Autodesk Inventor part; units mm, degrees
ref_plane "YZ Plane" through (0, 0, 0) normal (1, 0, 0) x (0, 1, 0)
ref_plane "XZ Plane" through (0, 0, 0) normal (0, 1, 0) x (-1, 0, 0)
ref_plane "XY Plane" through (0, 0, 0) normal (0, 0, 1) x (1, 0, 0)
sketch "Sketch1" plane through (0, 0, 0) normal (1, 0, 0) x (0, 1, 0)
  line L0 (-8.7654, 33.1522) -> (-8.7039, 33.1268)
  line L1 (8.7039, 33.1268) -> (8.7654, 33.1522)
  line L2 (-5, 27.5835) -> (-5, 0)
  line L3 (5, 27.5835) -> (5, 0)
  arc A0 (-5, 27.5835) -> (-8.7039, 33.1268) centre (-11, 27.5835) ccw
  arc A1 (8.7039, 33.1268) -> (5, 27.5835) centre (11, 27.5835) ccw
  line L4 (-7, 36) -> (7, 36)
  line L5 (-10, 36) -> (-10, 35)
  line L6 (10, 36) -> (10, 35)
  circle A2 centre (0, 0) radius 46 construction
  arc A3 (-10, 35) -> (-8.7654, 33.1522) centre (-8, 35) ccw
  arc A4 (8.7654, 33.1522) -> (10, 35) centre (8, 35) ccw
  circle A5 centre (0, 0) radius 1.5
  arc A6 (-5, 0) -> (5, 0) centre (0, 0) ccw
  line L7 (0, 0) -> (0, 36) construction
  line L8 (-10, 36) -> (-9.7321, 36)
  line L9 (10, 42) -> (-10, 42)
  line L10 (-10, 42) -> (-10, 36)
  line L11 (10, 36) -> (9.7321, 36)
  line L12 (10, 42) -> (10, 36)
  line L13 (-7, 36) -> (-7, 39)
  line L14 (-7, 39) -> (7, 39)
  line L15 (7, 39) -> (7, 36)
  point P0 (-5, 31.5926)
  point P1 (5, 31.5926)
  dimension "d25" = 10
  dimension "d32" = 6
  dimension "d33" = 6
  dimension "d82" = 46
  dimension "d90" = 2
  dimension "d93" = 1
  dimension "d95" = 22.5
  dimension "d109" = 3
  dimension "d112" = 36
  dimension "d113" = 5
  dimension "d115" = 20
  dimension "d118" = 6
  dimension "d120" = 6
extrude "Extrusion10" add sketch "Sketch1" along normal blind 3
fillet "Fillet1" radius 2 2 edges at (1.5, -10, 42) (1.5, 10, 42)
properties part number "27030914CameraMountA-2"
Input: part model. Units: mm. Frame: model coordinates. A direction names the side the tool comes from. Give positions to 0.01 mm unless a question says otherwise; leave off trailing zeros. Order: outer loops, then holes, each group sorted by start corner. A loop starts at its lowest first (then second) coordinate and runs counter-clockwise, first axis right, second up.
1. Section C-C on z = 7. Return the cut outline in (x, y).
Derived:
outline: (0, -5) - (3, -5) - (3, 5) - (0, 5) - close
2. Reachability of faces 1 (the flat face through (1, 0, 36)), 2 (the flat face through (1, 10, 38)), 3 (the flat face through (1, 5, 14)), 4 (the flat face through (1, -5, 14)) from +Z, -Z, +X, -X, +Y, -Y: full face, straight path, thin tool, end or side. Return the list, or none.
Derived:
face 1: +X, -X
face 2: +Z, -Z, +X, -X, +Y
face 3: -Z, +X, -X, +Y
face 4: -Z, +X, -X, -Y
3. Material intervals for L1, parallel to Z at x = 2.15, y = 0; L2, parallel to Y at x = 1.75, z = 27; L3, parallel to Y at x = 2, z = 34, sorted ascending.
Derived:
L1: z = -5 to -1.5, 1.5 to 36, 39 to 42
L2: y = -5 to 5
L3: y = -9.73 to 9.73
4. Section D-D on y = 7.5. Return the cut outline in (x, z).
Derived:
outline: (0, 32.46) - (3, 32.46) - (3, 42) - (0, 42) - close
5. Mould query, pull axis Y, two halves, no side actions, for faces 5 (the flat face through (3, 0, 24)), 6 (the cylindrical face through (1, 0, -5)), 7 (the flat face through (1, -7, 37)), 8 (the flat face through (1, -10, 38)). Classes: released by +Y, released by -Y, zero draft, split by the parting line, or undercut.
Derived:
face 5: zero draft
face 6: split by the parting line
face 7: undercut
face 8: released by -Y
6. Section B-B on x = 1.9. Return the cut outline in (y, z).
Derived:
outline: (-10, 35) arc R2 ccw to (-8.77, 33.15) - (-8.7, 33.13) arc R6 cw to (-5, 27.58) - (-5, 0) arc R5 ccw to (5, 0) - (5, 27.58) arc R6 cw to (8.7, 33.13) - (8.77, 33.15) arc R2 ccw to (10, 35) - (10, 40) arc R2 ccw to (8, 42) - (-8, 42) arc R2 ccw to (-10, 40) - close; hole (-7, 36) - (7, 36) - (7, 39) - (-7, 39) - close; hole circle Ø3 at (0, 0)
7. Section A-A on y = 0. Return the cut outline in (x, z), and give its area (3 significant figures).
Derived:
outline: (0, -5) - (3, -5) - (3, -1.5) - (0, -1.5) - close; (0, 1.5) - (3, 1.5) - (3, 36) - (0, 36) - close; (0, 39) - (3, 39) - (3, 42) - (0, 42) - close
area: 123 mm2
8. Pin query (flat end, axial travel): pin 1 (0.9 mm diameter, centred on x = 1, z = 13, fed in from +Y). Return the tip coordinate at first contact, or that it passes through.
Derived:
pin 1: stops at y = 5
